Here's how the part is built. I have some questions about the finished solid (model axes, mm). A direction names the side the tool comes from. Coordinates: 2 decimals unless noted, no trailing zeros. Write each loop counter-clockwise with the first axis right and the second up, starting at its lowest first coordinate (ties: lowest second). Pieces come first, ordered by that corner, then holes. Notation, with made-up numbers: M -33.5,-31 L -27.5,-31 A18 ccw -27.5,-6 Z; hole C 24,37 d11. An arc over 180 degrees is marked long. Write each question's results on one line, items separated by ' | '. Start each with the question number.
from build123d import *

# Parameters (mm, degrees)
F0_R     = 104
F0_R_2   = 68.5
F1_DEPTH = 19
F2_R     = 80
F2_R_2   = 74.5
F3_DEPTH = 5
F4_R     = 80
F5_DEPTH = 12
F6_SIZE2 = 1.1547005384
F6_SIZE  = 2
F7_R     = 4.99999
F9_D     = 14
F9_DEPTH = 25.5
F9_TIP   = 4.2060243332


# Not quite as in the source:
# - a fillet or chamfer is up to 0.001 mm smaller than in the source, because OpenCascade refuses the exact size


with BuildPart() as f1:
    # F0 (on Right) → F1 (new body)
    with BuildSketch(Plane.YZ):
        Circle(F0_R)
        Circle(F0_R_2, mode=Mode.SUBTRACT)
    extrude(amount=-F1_DEPTH)

    # F2 (on face) → F3 (join)
    with BuildSketch(Plane.YZ):
        Circle(F2_R)
        Circle(F2_R_2, mode=Mode.SUBTRACT)
    extrude(amount=F3_DEPTH)

    # F4 (on face) → F5 (cut)
    with BuildSketch(Plane(origin=(-19, 0, 0), x_dir=(0, -1, 0), z_dir=(-1, 0, 0))):
        Circle(F4_R)
    extrude(amount=-F5_DEPTH, mode=Mode.SUBTRACT)

    # F6
    f6_edges = [f1.edges().sort_by_distance(p)[0] for p in [
        (5, -80, 0),
    ]]
    f6_side = f1.faces().sort_by_distance((2.5, -80, 0))[0]
    chamfer(f6_edges, length=F6_SIZE, length2=F6_SIZE2, reference=f6_side)

    # F7 (radius 5 in the source; OpenCascade refuses exactly that, so slightly less here)
    f7_edges = [f1.edges().sort_by_distance(p)[0] for p in [
        (0, -74.5, 0),
    ]]
    fillet(f7_edges, radius=F7_R)

    # F9
    with Locations(Plane(origin=(-19, 0, 0), x_dir=(0, -1, 0), z_dir=(-1, 0, 0))):
        with Locations((0, -93), (-93, 0), (0, 93), (93, 0)):
            Hole(F9_D / 2, depth=F9_DEPTH)
            with Locations((0, 0, -(F9_DEPTH + F9_TIP / 2))):  # 118° drill point
                Cone(0, F9_D / 2, F9_TIP, mode=Mode.SUBTRACT)


solid = f1.part
1) I want a section at B-B, the plane x = -13.5. Write out the boundary of the cut face in (y, z).
2) Please list where these lines run through material, in increasing order: line 1 (Z direction, x = -13.25, y = 0); line 2 (X direction, y = -10, z = 91); line 3 (Y direction, x = -4.5, z = -25) (3 decimals). Write a range as [from, to].
3) For faces 4 (the flat face through (5, -47, -58)), 5 (the flat face through (0, -78, 24)), 6 (the cylindrical face through (-13.08, 17.34, -78.1)), which set-ups out of +Z, -Z, +X, -X, +Y, -Y let a thin tool reach every point of the face, with its end or its side?
4) I want a section at A-A, the plane z = 0. Give the number of separate pieces and of enclosed holes in the cut face, then the cut area to 3 significant figures.
5) I want a section at C-C, the plane y = -93. Write out the boundary of the cut face in (x, z), then the cut area to 3 significant figures.
6) For pin 1 Ø10 at (x, z) = (-16.5, 18.5) entering from -Y; pin 2 Ø1.5 at (x, y) = (-2, -24) entering from -Z; pin 3 Ø3 at (x, y) = (-7.5, 40) entering from -Z; pin 4 Ø12.5 at (y, z) = (-93, 0) entering from +X, each with a flat end and sliding along its axis, tell me the tip position at first contact or that it passes through.
7) We'd pull the mould along Y, two halves only. Please class faces 1 (the cylindrical face through (-9.37, -0.91, 99.94)), 2 (the cylindrical face through (-9.367, -82.531, -63.282)), 3 (the flat face through (-19, -78, 24)): pulls with the +Y half, pulls with the -Y half, needs draft (parallel to the pull), parting line crosses it, or undercut.
Output:
1) outline: C 0,0 d208; hole C -93,0 d14; hole C 0,0 d160; hole C 0,-93 d14; hole C 0,93 d14; hole C 93,0 d14
2) line 1: z = [-104, -100], [-86, -80], [80, 86], [100, 104] | line 2: x = [-19, 0] | line 3: y = [-100.95, -63.775], [63.775, 100.95]
3) face 4: +Z, -Z, +X, +Y, -Y | face 5: +X | face 6: -X
4) separate pieces: 4 | enclosed holes: 0 | area: 604 mm2
5) outline: M -19,-46.55 L 0,-46.55 L 0,-7 L -19,-7 Z; M -19,7 L 0,7 L 0,46.55 L -19,46.55 Z | area: 1,500 mm2
6) pin 1: stops at y = -103.12 | pin 2: stops at z = -101.37 | pin 3: stops at z = -96.61 | pin 4: passes through
7) face 1: undercut | face 2: parting line crosses it | face 3: needs draft
